```python
from build123d import *

# Parameters (mm, degrees)
SKETCH1_W                      = 235
SKETCH1_H                      = 1
BASE_FLANGE1_DEPTH             = 145
EDGE_FLANGE2_STRIP_W           = 24
EDGE_FLANGE2_STRIP_H           = 1
EDGE_FLANGE2_STRIP_CUT_DEPTH   = 290
EDGE_FLANGE2_STRIP_2_W         = 24
EDGE_FLANGE2_STRIP_2_H         = 1
EDGE_FLANGE2_STRIP_CUT_2_DEPTH = 290
EDGE_FLANGE2_DEPTH             = 290
EDGE_FLANGE2_BEND_DEPTH        = 290
EDGE_FLANGE3_STRIP_W           = 9
EDGE_FLANGE3_STRIP_H           = 1
EDGE_FLANGE3_STRIP_CUT_DEPTH   = 290
EDGE_FLANGE3_STRIP_2_W         = 9
EDGE_FLANGE3_STRIP_2_H         = 1
EDGE_FLANGE3_STRIP_CUT_2_DEPTH = 290
EDGE_FLANGE3_DEPTH             = 290
EDGE_FLANGE3_BEND_DEPTH        = 290
CUT_EXTRUDE1_START             = -10
CUT_EXTRUDE1_DEPTH             = 10


# Read off the part's stored shape, not the designer's step: Cut-Extrude1
# Sheet-metal steps are written as plain solids
with BuildPart() as part:
    # Sketch1 → Base-Flange1 (new, symmetric)
    with BuildSketch(Plane(origin=(0, 0, 0), x_dir=(1, 0, 0), z_dir=(0, 1, 0))):
        with Locations((0, -0.5)):
            Rectangle(SKETCH1_W, SKETCH1_H)
    extrude(amount=BASE_FLANGE1_DEPTH, both=True)

    # Edge-Flange2 strip (across the edge) → Edge-Flange2 strip cut (cut)
    with BuildSketch(Plane(origin=(-117.5, 145, 1), x_dir=(1, 0, 0), z_dir=(0, -1, 0))):
        with Locations((-1, -0.5)):
            Rectangle(EDGE_FLANGE2_STRIP_W, EDGE_FLANGE2_STRIP_H)
    extrude(amount=EDGE_FLANGE2_STRIP_CUT_DEPTH, mode=Mode.SUBTRACT)

    # Edge-Flange2 strip 2 (across the edge) → Edge-Flange2 strip cut 2 (cut)
    with BuildSketch(Plane(origin=(117.5, -145, 1), x_dir=(-1, 0, 0), z_dir=(0, 1, 0))):
        with Locations((-1, -0.5)):
            Rectangle(EDGE_FLANGE2_STRIP_2_W, EDGE_FLANGE2_STRIP_2_H)
    extrude(amount=EDGE_FLANGE2_STRIP_CUT_2_DEPTH, mode=Mode.SUBTRACT)

    # Edge-Flange2 section (across the edge) → Edge-Flange2 (add)
    with BuildSketch(Plane(origin=(-117.5, 145, 1), x_dir=(1, 0, 0), z_dir=(0, -1, 0))):
        with BuildLine():
            Line((0, 10), (0, 130.826439119))
            Line((0, 130.826439119), (1, 130.826439119))
            Line((1, 130.826439119), (1, 10))
            ThreePointArc((1, 10), (3.928932188, 2.928932188), (11, 0))
            Line((11, 0), (11, -1))
            ThreePointArc((11, -1), (3.221825407, 2.221825407), (0, 10))
        make_face()
    extrude(amount=EDGE_FLANGE2_DEPTH)

    # Edge-Flange2 section 2 (across the edge) → Edge-Flange2 bend (add)
    with BuildSketch(Plane(origin=(117.5, -145, 1), x_dir=(-1, 0, 0), z_dir=(0, 1, 0))):
        with BuildLine():
            Line((0, 10), (0, 130.826439119))
            Line((0, 130.826439119), (1, 130.826439119))
            Line((1, 130.826439119), (1, 10))
            ThreePointArc((1, 10), (3.928932188, 2.928932188), (11, 0))
            Line((11, 0), (11, -1))
            ThreePointArc((11, -1), (3.221825407, 2.221825407), (0, 10))
        make_face()
    extrude(amount=EDGE_FLANGE2_BEND_DEPTH)

    # Edge-Flange3 strip (across the edge) → Edge-Flange3 strip cut (cut)
    with BuildSketch(Plane(origin=(-116.5, 145, 131.826439119), x_dir=(0, 0, -1), z_dir=(0, -1, 0))):
        with Locations((-1, -0.5)):
            Rectangle(EDGE_FLANGE3_STRIP_W, EDGE_FLANGE3_STRIP_H)
    extrude(amount=EDGE_FLANGE3_STRIP_CUT_DEPTH, mode=Mode.SUBTRACT)

    # Edge-Flange3 strip 2 (across the edge) → Edge-Flange3 strip cut 2 (cut)
    with BuildSketch(Plane(origin=(116.5, -145, 131.826439119), x_dir=(0, 0, -1), z_dir=(0, 1, 0))):
        with Locations((-1, -0.5)):
            Rectangle(EDGE_FLANGE3_STRIP_2_W, EDGE_FLANGE3_STRIP_2_H)
    extrude(amount=EDGE_FLANGE3_STRIP_CUT_2_DEPTH, mode=Mode.SUBTRACT)

    # Edge-Flange3 section (across the edge) → Edge-Flange3 (add)
    with BuildSketch(Plane(origin=(-116.5, 145, 131.826439119), x_dir=(0, 0, -1), z_dir=(0, -1, 0))):
        with BuildLine():
            Line((0, 2.5), (0, 16))
            Line((0, 16), (1, 16))
            Line((1, 16), (1, 2.5))
            ThreePointArc((1, 2.5), (1.732233047, 0.732233047), (3.5, 0))
            Line((3.5, 0), (3.5, -1))
            ThreePointArc((3.5, -1), (1.025126266, 0.025126266), (0, 2.5))
        make_face()
    extrude(amount=EDGE_FLANGE3_DEPTH)

    # Edge-Flange3 section 2 (across the edge) → Edge-Flange3 bend (add)
    with BuildSketch(Plane(origin=(116.5, -145, 131.826439119), x_dir=(0, 0, -1), z_dir=(0, 1, 0))):
        with BuildLine():
            Line((0, 2.5), (0, 16))
            Line((0, 16), (1, 16))
            Line((1, 16), (1, 2.5))
            ThreePointArc((1, 2.5), (1.732233047, 0.732233047), (3.5, 0))
            Line((3.5, 0), (3.5, -1))
            ThreePointArc((3.5, -1), (1.025126266, 0.025126266), (0, 2.5))
        make_face()
    extrude(amount=EDGE_FLANGE3_BEND_DEPTH)

    # Cut-Extrude1 outline → Cut-Extrude1 (cut)
    with BuildSketch(Plane(origin=(0, 145, 0), x_dir=(1, 0, 0), z_dir=(0, 1, 0)).offset(CUT_EXTRUDE1_START)):
        with BuildLine():
            ThreePointArc((114, -131.826439119), (116.474873734, -130.801312853), (117.5, -128.326439119))
            Line((117.5, -128.326439119), (116.5, -128.326439119))
            ThreePointArc((116.5, -128.326439119), (115.767766953, -130.094206072), (114, -130.826439119))
            Line((114, -130.826439119), (100.5, -130.826439119))
            Line((100.5, -130.826439119), (100.5, -131.826439119))
            Line((100.5, -131.826439119), (114, -131.826439119))
        make_face()
        with BuildLine():
            ThreePointArc((-114, -130.826439119), (-115.767766953, -130.094206072), (-116.5, -128.326439119))
            Line((-116.5, -128.326439119), (-117.5, -128.326439119))
            ThreePointArc((-117.5, -128.326439119), (-116.474873734, -130.801312853), (-114, -131.826439119))
            Line((-114, -131.826439119), (-100.5, -131.826439119))
            Line((-100.5, -131.826439119), (-100.5, -130.826439119))
            Line((-100.5, -130.826439119), (-114, -130.826439119))
        make_face()
    extrude(amount=CUT_EXTRUDE1_DEPTH, mode=Mode.SUBTRACT)


solid = part.part
```
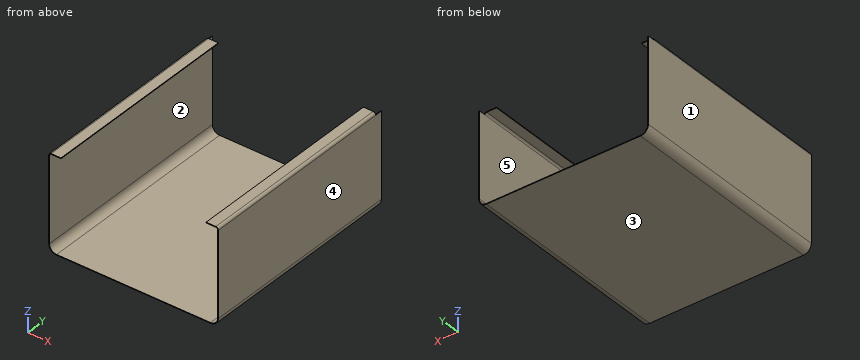
Design review of the part built by this model. Coordinates are the model's own, in mm. Face numbers are marked on the shaded views. A direction names the side the tool comes from. Coordinates: 2 decimals unless noted, no trailing zeros. Order: outer loops, then holes, each group sorted by start corner. A loop starts at its lowest first (then second) coordinate and runs counter-clockwise, first axis right, second up. Notation, with made-up numbers: (19.25, 16) -> (45.25, 16) arc R17 cw to (45.25, 32) -> close; hole circle Ø6 at (43, -39). An arc over 180 degrees is marked (long way). One line per item, written item: value. Start each with the question number.
Q1. Take a section at A-A, the plane z = 60. State the section outline as (x, y) points.
Q2. Take a section at C-C, the plane x = -87. State the section outline as (y, z) points.
Q3. Insertion check: pin 1 Ø3 at (x, y) = (-37, 81) entering from -Z; pin 2 Ø0.8 at (y, z) = (26.5, 131.5) entering from +X; pin 3 Ø1.5 at (x, y) = (-30, 95.5) entering from +Z; pin 4 Ø0.5 at (x, y) = (-117, 141) entering from +Z. Each pin has a flat end and moves straight along its axis. Give the tip position at first contact, or say it passes through.
Q4. Mouldability with a two-part tool opening along X and no side actions: class the marked faces 3, 4 and 5 as pulls with the +X half, pulls with the -X half, needs draft (parallel to the pull), parting line crosses it, or undercut.
Q5. Take a section at B-B, the plane y = -15. State the section outline as (x, z) points, then the cut area to 3 significant figures.
Q6. Tool access review of the marked faces 1 and 2: name each direction out of +Z, -Z, +X, -X, +Y, -Y from which nothing blocks a thin tool from reaching the whole face with its end or side.
Q7. For probe 1 along X at (y, z) = (19, 25); probe 2 along Z at (x, y) = (37, 48.5), list the stretches that pass through material, from the lowest coordinate up.
Values follow:
1. outline: (-117.5, -145) -> (-116.5, -145) -> (-116.5, 145) -> (-117.5, 145) -> close; (116.5, -145) -> (117.5, -145) -> (117.5, 145) -> (116.5, 145) -> close
2. outline: (-145, 0) -> (145, 0) -> (145, 1) -> (-145, 1) -> close
3. pin 1: stops at z = 0
3. pin 2: stops at x = 116.13
3. pin 3: stops at z = 1
3. pin 4: stops at z = 128.33
4. face 3: needs draft
4. face 4: pulls with the +X half
4. face 5: undercut
5. outline: (-117.5, 11) arc R11 ccw to (-106.5, 0) -> (106.5, 0) arc R11 ccw to (117.5, 11) -> (117.5, 128.33) arc R3.5 ccw to (114, 131.83) -> (100.5, 131.83) -> (100.5, 130.83) -> (114, 130.83) arc R2.5 cw to (116.5, 128.33) -> (116.5, 11) arc R10 cw to (106.5, 1) -> (-106.5, 1) arc R10 cw to (-116.5, 11) -> (-116.5, 128.33) arc R2.5 cw to (-114, 130.83) -> (-100.5, 130.83) -> (-100.5, 131.83) -> (-114, 131.83) arc R3.5 ccw to (-117.5, 128.33) -> close
5. area: 517 mm2
6. face 1: +Z, -Z, -X, +Y, -Y
6. face 2: +Y, -Y
7. probe 1: x = -117.5 to -116.5, 116.5 to 117.5
7. probe 2: z = 0 to 1
